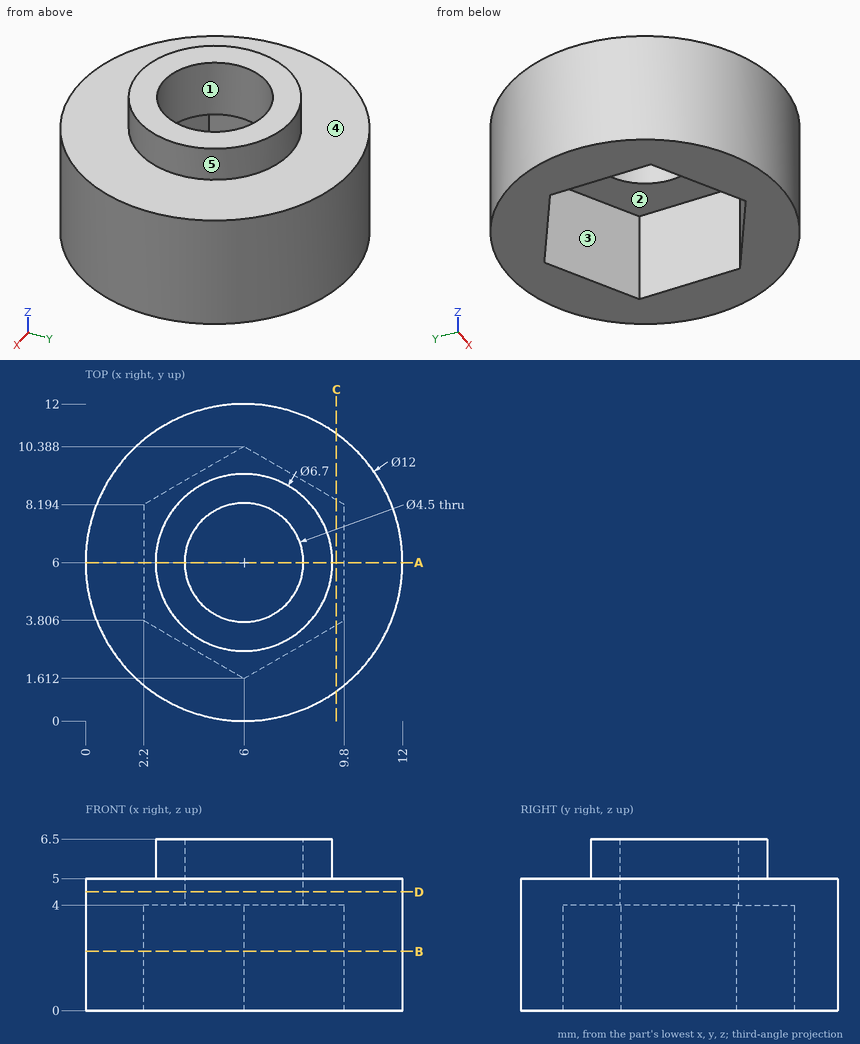
Verification items for this drawing (mm, ordinates from the low corner). A direction names the side the tool comes from. Coordinates: 2 decimals unless noted, no trailing zeros. Write each loop counter-clockwise with the first axis right and the second up, starting at its lowest first coordinate (ties: lowest second). Pieces come first, ordered by that corner, then holes. Notation, with made-up numbers: M -35,43.25 L -9,43.25 A10 ccw -9,60.25 Z; hole C 41,12 d8. An arc over 180 degrees is marked long. One line per item, written item: value. Start each with the question number.
(1) Sectioned sample at D-D, the plane z = 4.5. Enter the section's corners in (x, y).
(2) Tool access check on the marked faces 1 and 2. Record the directions out of +Z, -Z, +X, -X, +Y, -Y that give a thin tool (end or side, any length) a straight path to the whole face; none if there is none.
(3) Sectioned sample at A-A, the plane y = 6. Enter the section's corners in (x, z).
(4) Scan lines: line 1 along Y through (x, z) = (6, 5.1); line 2 along Z through (x, y) = (8.75, 3.25); line 3 along Z through (x, y) = (8, 10). Record each from-to range of solid material in increasing order. Write a range as [from, to].
(5) Release check for a two-part mould opening along Y. For the marked faces 3, 4 and 5 record: released by +Y, released by -Y, zero draft, split by the parting line, or undercut.
(6) Sectioned sample at C-C, the plane x = 9.5. Enter the section's corners in (y, z), and give its area (3 significant figures).
(7) Sectioned sample at B-B, the plane z = 2.25. Enter the section's corners in (x, y), and give its area (3 significant figures).
Filled sheet:
1. outline: C 6,6 d12; hole C 6,6 d4.5
2. face 1: +Z, -Z
2. face 2: -Z
3. outline: M 0,0 L 2.2,0 L 2.2,4 L 3.75,4 L 3.75,6.5 L 2.65,6.5 L 2.65,5 L 0,5 Z; M 8.25,4 L 9.8,4 L 9.8,0 L 12,0 L 12,5 L 9.35,5 L 9.35,6.5 L 8.25,6.5 Z
4. line 1: [2.65, 3.75], [8.25, 9.35]
4. line 2: [4, 5]
4. line 3: [0, 5]
5. face 3: undercut
5. face 4: zero draft
5. face 5: split by the parting line
6. outline: M 1.13,0 L 3.63,0 L 3.63,4 L 8.37,4 L 8.37,0 L 10.87,0 L 10.87,5 L 1.13,5 Z
6. area: 29.8 mm²
7. outline: C 6,6 d12; hole M 2.2,3.81 L 6,1.61 L 9.8,3.81 L 9.8,8.19 L 6,10.39 L 2.2,8.19 Z
7. area: 63.1 mm²
